```python
from build123d import *

# Parameters (mm, degrees)
SKETCH_1_R          = 1.75
EXTRUDE_1_DEPTH     = 5.9
CUT_EXTRUDE_1_DEPTH = 2.5


with BuildPart() as part:
    # 草图1 → 凸台-拉伸1 (new body)
    with BuildSketch(Plane.XY):
        with BuildLine():
            Line((-11.25, 16.25), (-11.25, -16.25))
            ThreePointArc((-11.25, -16.25), (-9.785533906, -19.785533906), (-6.25, -21.25))
            Line((-6.25, -21.25), (6.25, -21.25))
            ThreePointArc((6.25, -21.25), (9.785533906, -19.785533906), (11.25, -16.25))
            Line((11.25, -16.25), (11.25, -11.05))
            ThreePointArc((11.25, -11.05), (9.785533906, -7.514466094), (6.25, -6.05))
            Line((6.25, -6.05), (0, -6.05))
            ThreePointArc((0, -6.05), (-6.05, 0), (0, 6.05))
            Line((0, 6.05), (6.25, 6.05))
            ThreePointArc((6.25, 6.05), (9.785533906, 7.514466094), (11.25, 11.05))
            Line((11.25, 11.05), (11.25, 16.25))
            ThreePointArc((11.25, 16.25), (9.785533906, 19.785533906), (6.25, 21.25))
            Line((6.25, 21.25), (-6.25, 21.25))
            ThreePointArc((-6.25, 21.25), (-9.785533906, 19.785533906), (-11.25, 16.25))
        make_face()
        with Locations((0, 16.25)):
            Circle(SKETCH_1_R, mode=Mode.SUBTRACT)
        with Locations((0, -16.25)):
            Circle(SKETCH_1_R, mode=Mode.SUBTRACT)
    extrude(amount=EXTRUDE_1_DEPTH)

    # 草图2 → 切除-拉伸1 (cut)
    with BuildSketch(Plane(origin=(0, 0, 0), x_dir=(-1, 0, 0), z_dir=(0, 0, -1))):
        Polygon((1.645448267, 13.4), (3.290896534, 16.25), (1.645448267, 19.1), (-1.645448267, 19.1), (-3.290896534, 16.25), (-1.645448267, 13.4), align=None)
        Polygon((-1.645448267, -13.4), (-3.290896534, -16.25), (-1.645448267, -19.1), (1.645448267, -19.1), (3.290896534, -16.25), (1.645448267, -13.4), align=None)
    extrude(amount=-CUT_EXTRUDE_1_DEPTH, mode=Mode.SUBTRACT)


solid = part.part
```
Design review of the part built by this model. Coordinates are the model's own, in mm. A direction names the side the tool comes from. Give positions to 0.01 mm unless a question says otherwise; leave off trailing zeros. Order: outer loops, then holes, each group sorted by start corner. A loop starts at its lowest first (then second) coordinate and runs counter-clockwise, first axis right, second up. Notation, with made-up numbers: (15, -39) -> (25, -39) arc R24 cw to (25, 0) -> close; hole circle Ø8 at (-3, -21.5). An arc over 180 degrees is marked (long way). Write each question's results on one line, items separated by ' | '. Start each with the question number.
Q1. Add section A-A on z = 4.1. Give the boundary of the cut face in (x, y).
Q2. Add section B-B on x = -0.75. Give the boundary of the cut face in (y, z), and give its area (3 significant figures).
Q3. Add section C-C on z = 1.5. Give the boundary of the cut face in (x, y), and give its area (3 significant figures).
Q4. Machinability: for faces 1 (the flat face through (-1.4, -14.9, 2.5)), 2 (the cylindrical face through (9.75, -19.82, 2.91)), which of the approach directions +Z, -Z, +X, -X, +Y, -Y give a long, thin tool a straight path to every point of the face, cutting with its end or side? Answer none if there is none.
Q5. Wall thickness on L1, parallel to X at y = 16.25, z = 3.55; L2, parallel to Y at x = 2, z = 3.85: over which ranges is each line inside the solid? List them lowest first. Write a range as from..to.
Q6. Add section D-D on y = 0. Give the boundary of the cut face in (x, z).
Q7. For pin 1 (6.5 mm diameter, centred on x = 1, y = 17.5, fed in from -Z); pin 2 (1 mm diameter, centred on y = 1, z = 5, fed in from +X), all flat-tipped, find the tip position at first contact; note any pin that passes through.
Q8. Mouldability with a two-part tool opening along X and no side actions: class faces 3 (the cylindrical face through (9.75, 7.48, 2.91)), 4 (the flat face through (-5, 5, 0)), 5 (the flat face through (-1, 18, 2.5)), 6 (the flat face through (-2.48, 17.655, 1.232)) as +X half, -X half, draft (parallel to the pull), parting line (faces both ways), or undercut.
Found:
1) outline: (-11.25, -16.25) arc R5 ccw to (-6.25, -21.25) -> (6.25, -21.25) arc R5 ccw to (11.25, -16.25) -> (11.25, -11.05) arc R5 ccw to (6.25, -6.05) -> (0, -6.05) arc R6.05 cw to (0, 6.05) -> (6.25, 6.05) arc R5 ccw to (11.25, 11.05) -> (11.25, 16.25) arc R5 ccw to (6.25, 21.25) -> (-6.25, 21.25) arc R5 ccw to (-11.25, 16.25) -> close; hole circle Ø3.5 at (0, -16.25); hole circle Ø3.5 at (0, 16.25)
2) outline: (-21.25, 0) -> (-19.1, 0) -> (-19.1, 2.5) -> (-17.83, 2.5) -> (-17.83, 5.9) -> (-21.25, 5.9) -> close; (-14.67, 2.5) -> (-13.4, 2.5) -> (-13.4, 0) -> (-6, 0) -> (-6, 5.9) -> (-14.67, 5.9) -> close; (6, 0) -> (13.4, 0) -> (13.4, 2.5) -> (14.67, 2.5) -> (14.67, 5.9) -> (6, 5.9) -> close; (17.83, 2.5) -> (19.1, 2.5) -> (19.1, 0) -> (21.25, 0) -> (21.25, 5.9) -> (17.83, 5.9) -> close | area: 130 mm2
3) outline: (-11.25, -16.25) arc R5 ccw to (-6.25, -21.25) -> (6.25, -21.25) arc R5 ccw to (11.25, -16.25) -> (11.25, -11.05) arc R5 ccw to (6.25, -6.05) -> (0, -6.05) arc R6.05 cw to (0, 6.05) -> (6.25, 6.05) arc R5 ccw to (11.25, 11.05) -> (11.25, 16.25) arc R5 ccw to (6.25, 21.25) -> (-6.25, 21.25) arc R5 ccw to (-11.25, 16.25) -> close; hole (-3.29, -16.25) -> (-1.65, -19.1) -> (1.65, -19.1) -> (3.29, -16.25) -> (1.65, -13.4) -> (-1.65, -13.4) -> close; hole (-3.29, 16.25) -> (-1.65, 13.4) -> (1.65, 13.4) -> (3.29, 16.25) -> (1.65, 19.1) -> (-1.65, 19.1) -> close | area: 674 mm2
4) face 1: -Z | face 2: +Z, -Z, +X, -Y
5) L1: x = -11.25..-1.75, 1.75..11.25 | L2: y = -21.25..-6.05, 6.05..21.25
6) outline: (-11.25, 0) -> (-6.05, 0) -> (-6.05, 5.9) -> (-11.25, 5.9) -> close
7) pin 1: stops at z = 0 | pin 2: stops at x = -5.86
8) face 3: +X half | face 4: draft | face 5: undercut | face 6: undercut
